Read the model definition and answer for the solid it produces. Units are mm, in the model's axes. Give positions to 0.01 mm unless a question says otherwise; leave off trailing zeros. Order: outer loops, then holes, each group sorted by start corner. A loop starts at its lowest first (then second) coordinate and runs counter-clockwise, first axis right, second up.
Item 1: A cutting plane is placed at B-B (z = -55). Write down the section's boundary in (x, y), plus the area to 3 significant figures.
Item 2: A cutting plane is placed at A-A (y = 0). Write down the section's boundary in (x, z).
Item 3: Given pin 1 Ø4.5 at (y, z) = (20.5, 1.5) entering from +X; pin 2 Ø3.5 at (x, y) = (0, 0) entering from -Z; pin 3 Ø4.5 at (y, z) = (21, -2.5) entering from -X, each flat-ended and moving along its own axis, determine where each tip first touches the part or whether it passes through.
Item 4: A cutting plane is placed at D-D (z = 19). Write down the section's boundary in (x, y).
Item 5: A cutting plane is placed at C-C (y = 20). Write down the section's boundary in (x, z).
Item 6: Find the intervals of material crossed by line 1 along Y through (x, z) = (0, -56); line 2 along Z through (x, y) = (-2, -2); line 3 along Z through (x, y) = (4, 17.5), in increasing order.
from build123d import *

# Parameters (mm, degrees)
BOSS_EXTRUDE2_DEPTH      = 65
BOSS_EXTRUDE2_DEPTH_BACK = 65
SKETCH1_R                = 17.5
BOSS_EXTRUDE3_DEPTH      = 5
BOSS_EXTRUDE3_DEPTH_BACK = 5
SKETCH2_W                = 10
SKETCH2_H                = 10
SKETCH3_R                = 3
CUT_EXTRUDE1_DEPTH       = 15
SKETCH4_R                = 1
CUT_EXTRUDE2_DEPTH       = 10


with BuildPart() as part:
    # Sketch1 → Boss-Extrude2 (new, two sides: drawn at the far end of the back side and taken through both)
    with BuildSketch(Plane.XY.offset(-BOSS_EXTRUDE2_DEPTH_BACK)):
        Circle(SKETCH1_R)
    extrude(amount=BOSS_EXTRUDE2_DEPTH + BOSS_EXTRUDE2_DEPTH_BACK)

    # Sketch2 → Boss-Extrude3 (add, two sides: drawn at the far end of the back side and taken through both)
    with BuildSketch(Plane.XY.offset(-BOSS_EXTRUDE3_DEPTH_BACK)):
        with Locations((0.175667468, 17.49911829)):
            Rectangle(SKETCH2_W, SKETCH2_H)
    extrude(amount=BOSS_EXTRUDE3_DEPTH + BOSS_EXTRUDE3_DEPTH_BACK)

    # Sketch3 → Cut-Extrude1 (cut)
    with BuildSketch(Plane.XY.offset(65)):
        Circle(SKETCH3_R)
    cut_extrude1 = extrude(amount=-CUT_EXTRUDE1_DEPTH, mode=Mode.SUBTRACT)

    # Mirror1: Cut-Extrude1 across plane
    add(cut_extrude1.mirror(Plane.XY), mode=Mode.SUBTRACT)

    # Sketch4 → Cut-Extrude2 (cut)
    with BuildSketch(Plane(origin=(0, 22.49911829, 0), x_dir=(1, 0, 0), z_dir=(0, 1, 0))):
        with Locations(Location((0.175667468, -3.5, 0), (0, 0, 270))):
            Circle(SKETCH4_R)
    extrude(amount=-CUT_EXTRUDE2_DEPTH, mode=Mode.SUBTRACT)


solid = part.part
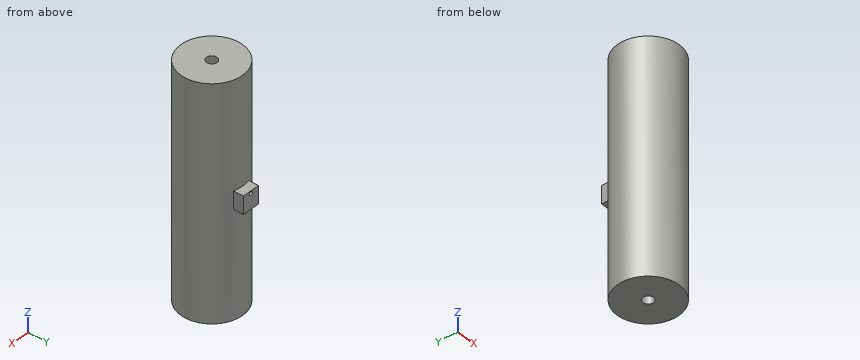
Response values:
1. outline: circle Ø35 at (0, 0); hole circle Ø6 at (0, 0)
1. area: 934 mm2
2. outline: (-17.5, -65) - (-3, -65) - (-3, -50) - (3, -50) - (3, -65) - (17.5, -65) - (17.5, 65) - (3, 65) - (3, 50) - (-3, 50) - (-3, 65) - (-17.5, 65) - close
3. pin 1: stops at x = 5.18
3. pin 2: stops at z = -50
3. pin 3: stops at x = -4.82
4. outline: circle Ø35 at (0, 0)
5. outline: (-4.82, -5) - (5.18, -5) - (5.18, 5) - (-4.82, 5) - close; hole circle Ø2 at (0.18, 3.5)
6. line 1: y = -17.5 to -3, 3 to 17.5
6. line 2: z = -50 to 50
6. line 3: z = -5 to 5
